Here's how the part is built. I have some questions about the finished solid (model axes, mm). Face numbers are marked on the shaded views. A direction names the side the tool comes from. Give positions to 0.01 mm unless a question says otherwise; leave off trailing zeros. Write each loop counter-clockwise with the first axis right and the second up, starting at its lowest first coordinate (ties: lowest second). Pieces come first, ordered by that corner, then holes. Notation, with made-up numbers: (-36.75, 5.25) - (4.25, 5.25) arc R26 cw to (4.25, 26.25) - close; hole circle Ø3 at (58.5, 39). An arc over 180 degrees is marked (long way). Write each question's results on one line, items separated by ' | '. Start each with the question number.
Item 1: Please list where these lines run through material, in increasing order: line 1 along X through (y, z) = (-11.25, 20); line 2 along Y through (x, z) = (4.5, 0.5); line 3 along Y through (x, z) = (0, 19.5).
Item 2: Which directions (+Z, -Z, +X, -X, +Y, -Y) give clear straight access to the entire face, cutting with the end or side of a thin tool? Please do the marked faces 1, 2 and 3.
Item 3: Suppose I cut it at D-D on x = 2.5. List the corners of the cut face in (y, z) for me, then the cut area to 3 significant figures.
Item 4: Suppose I cut it at B-B on z = 24. List the corners of the cut face in (x, y) for me.
Item 5: Suppose I cut it at A-A on y = -1.5. List the corners of the cut face in (x, z) for me, then the cut area to 3 significant figures.
Item 6: Suppose I cut it at C-C on x = -3. List the corners of the cut face in (y, z) for me.
Item 7: Will these pins go through, and if not, where does the flat tip stop? P1, Ø10, axis at y = -5.5, z = 20, coming from the -X side; P2, Ø1, axis at x = 4, z = 3, coming from the +Y side; P3, Ø6.5, axis at y = -5, z = 21, coming from the +X side; P4, Ø4, axis at x = 6.5, y = -3.5, coming from the -Z side.
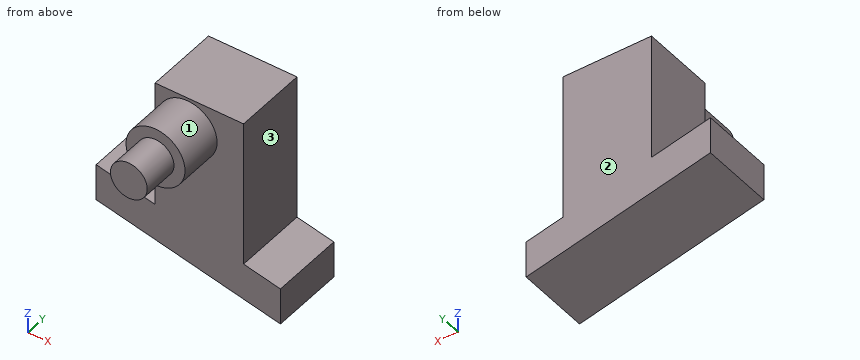
```python
from build123d import *

# Parameters (mm, degrees)
F1_DEPTH = 12.7
F2_R     = 5.08
F3_DEPTH = 7.62
F4_R     = 3.175
F5_DEPTH = 6.35


with BuildPart() as f1:
    # F0 (on Front) → F1 (new body)
    with BuildSketch(Plane.XZ):
        Polygon((-4.581327, 29.096584), (-4.581327, 7.100181), (10.658673, 3.696584), (10.658673, 29.096584), align=None)
        Polygon((-4.581327, 7.100181), (-14.741327, 9.369245), (-14.741327, 3.019245), (17.008673, -4.071582), (17.008673, 2.278418), (10.658673, 3.696584), align=None)
    extrude(amount=F1_DEPTH)

    # F2 (on face) → F3 (join)
    with BuildSketch(Plane.XZ.offset(12.7)):
        with Locations((1.006673, 23.508584)):
            Circle(F2_R)
    extrude(amount=F3_DEPTH)

    # F4 (on face) → F5 (join)
    with BuildSketch(Plane.XZ.offset(20.32)):
        with Locations((1.006673, 23.508584)):
            Circle(F4_R)
    extrude(amount=F5_DEPTH)


solid = f1.part
```
Checked values:
1) line 1: x = -4.58 to 10.66 | line 2: y = -12.7 to 0 | line 3: y = -20.32 to 0
2) face 1: -Y | face 2: +Z, -Z, +X, -X, +Y | face 3: +Z, +X, +Y, -Y
3) outline: (-26.67, 20.71) - (-20.32, 20.71) - (-20.32, 18.65) - (-12.7, 18.65) - (-12.7, -0.83) - (0, -0.83) - (0, 29.1) - (-12.7, 29.1) - (-12.7, 28.36) - (-20.32, 28.36) - (-20.32, 26.31) - (-26.67, 26.31) - close | area: 490 mm^2
4) outline: (-4.58, -12.7) - (-4.05, -12.7) - (-4.05, -20.32) - (-2.13, -20.32) - (-2.13, -26.67) - (4.14, -26.67) - (4.14, -20.32) - (6.06, -20.32) - (6.06, -12.7) - (10.66, -12.7) - (10.66, 0) - (-4.58, 0) - close
5) outline: (-14.74, 3.02) - (17.01, -4.07) - (17.01, 2.28) - (10.66, 3.7) - (10.66, 29.1) - (-4.58, 29.1) - (-4.58, 7.1) - (-14.74, 9.37) - close | area: 563 mm^2
6) outline: (-20.32, 20.39) - (-12.7, 20.39) - (-12.7, 0.4) - (0, 0.4) - (0, 29.1) - (-12.7, 29.1) - (-12.7, 26.63) - (-20.32, 26.63) - close
7) P1: stops at x = -4.58 | P2: stops at y = 0 | P3: stops at x = 10.66 | P4: stops at z = -2.17
